Can you work these out from the model? Positions are in its coordinate system, mm. Face numbers are marked on the shaded views. Give positions to 0.01 mm unless a question says otherwise; leave off trailing zeros. Loops run counter-clockwise (first coordinate to the right, second up) from the corner with the lowest first, then second, coordinate; pieces in that order, holes last.
from build123d import *

# Parameters (mm, degrees)
SKETCH_1_W          = 120
SKETCH_1_H          = 135
EXTRUDE_1_DEPTH     = 4
SKETCH_2_W          = 7
SKETCH_2_H          = 95
EXTRUDE_2_DEPTH     = 11
SKETCH_4_R          = 2.35
CUT_EXTRUDE_2_DEPTH = 118.904622471
SKETCH_5_W          = 120
SKETCH_5_H          = 35
CUT_EXTRUDE_3_DEPTH = 10
FILLET_1_R          = 2


with BuildPart() as part:
    # 草图1 → 凸台-拉伸1 (new body)
    with BuildSketch(Plane(origin=(0, 0, 0), x_dir=(1, 0, 0), z_dir=(0, 1, 0))):
        Rectangle(SKETCH_1_W, SKETCH_1_H)
    extrude(amount=EXTRUDE_1_DEPTH)

    # 草图2 → 凸台-拉伸2 (add)
    with BuildSketch(Plane(origin=(0, 4, 0), x_dir=(1, 0, 0), z_dir=(0, 1, 0))):
        with Locations((-32, 20)):
            Rectangle(SKETCH_2_W, SKETCH_2_H)
        with Locations((32, 20)):
            Rectangle(SKETCH_2_W, SKETCH_2_H)
    extrude(amount=EXTRUDE_2_DEPTH)

    # 草图4 → 切除-拉伸2 (cut, through all)
    with BuildSketch(Plane.ZY.offset(35.5)):
        with Locations((20, 9)):
            Circle(SKETCH_4_R)
        with BuildLine():
            Line((-60, 11.35), (-20, 11.35))
            ThreePointArc((-20, 11.35), (-17.65, 9), (-20, 6.65))
            Line((-20, 6.65), (-60, 6.65))
            ThreePointArc((-60, 6.65), (-62.35, 9), (-60, 11.35))
        make_face()
    extrude(amount=-CUT_EXTRUDE_2_DEPTH, mode=Mode.SUBTRACT)

    # 草图5 → 切除-拉伸3 (cut)
    with BuildSketch(Plane(origin=(0, 4, 0), x_dir=(1, 0, 0), z_dir=(0, 1, 0))):
        with Locations((0, -50)):
            Rectangle(SKETCH_5_W, SKETCH_5_H)
    extrude(amount=-CUT_EXTRUDE_3_DEPTH, mode=Mode.SUBTRACT)

    # 圆角1
    fillet_1_edges = [part.edges().sort_by_distance(p)[0] for p in [
        (-35.5, 4, -20),
        (-32, 15, -67.5),
        (-32, 15, 27.5),
        (35.5, 4, -20),
        (32, 15, -67.5),
        (32, 15, 27.5),
        (-60, 2, -67.5),
        (60, 2, -67.5),
        (60, 2, 32.5),
        (-60, 2, 32.5),
    ]]
    fillet(fillet_1_edges, radius=FILLET_1_R)


solid = part.part
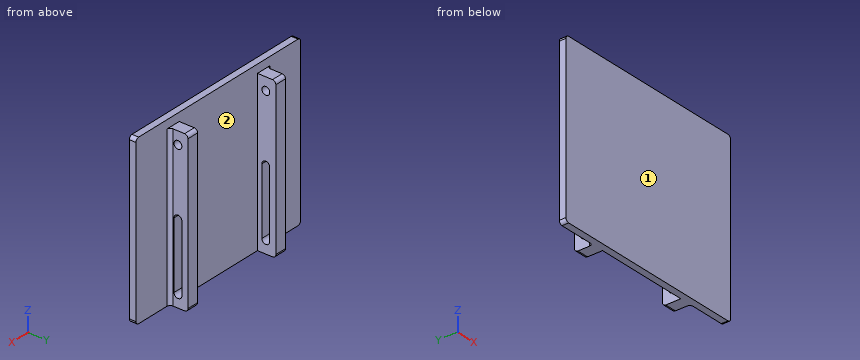
(1) Please list where these lines run through material, in increasing order: probe 1 along Y at (x, z) = (-34, 20); probe 2 along X at (y, z) = (12, -46); probe 3 along Z at (x, y) = (-30, 10).
Returned:
probe 1: y = 0 to 6.65, 11.35 to 15
probe 2: x = -35.5 to -28.5, 28.5 to 35.5
probe 3: z = -67.5 to -62.13, -17.87 to 17.87, 22.13 to 27.5
(2) Suppose I cut it at D-D on x = 27. List the corners of the cut face in (y, z) for me.
Returned:
outline: (0, -67.5) - (4, -67.5) - (4, 32.5) - (0, 32.5) - close
(3) Thinking about a two-plate mould opening in X: for the marked faces 1 and 2, which applies, pulls with the +X half, pulls with the -X half, needs draft (parallel to the pull), parting line crosses it, or undercut?
Returned:
face 1: needs draft
face 2: undercut
(4) Suppose I cut it at C-C on z = 9.5. List the corners of the cut face in (x, y) for me, plus the area to 3 significant figures.
Returned:
outline: (-60, 0) - (60, 0) - (60, 4) - (37.5, 4) arc R2 cw to (35.5, 6) - (35.5, 15) - (28.5, 15) - (28.5, 4) - (-28.5, 4) - (-28.5, 15) - (-35.5, 15) - (-35.5, 6) arc R2 cw to (-37.5, 4) - (-60, 4) - close
area: 636 mm2
(5) Suppose I cut it at B-B on z = 20. List the corners of the cut face in (x, y) for me, plus the area to 3 significant figures.
Returned:
outline: (-60, 0) - (60, 0) - (60, 4) - (37.5, 4) arc R2 cw to (35.5, 6) - (35.5, 6.65) - (28.5, 6.65) - (28.5, 4) - (-28.5, 4) - (-28.5, 6.65) - (-35.5, 6.65) - (-35.5, 6) arc R2 cw to (-37.5, 4) - (-60, 4) - close; (-35.5, 11.35) - (-28.5, 11.35) - (-28.5, 15) - (-35.5, 15) - close; (28.5, 11.35) - (35.5, 11.35) - (35.5, 15) - (28.5, 15) - close
area: 570 mm2
(6) Will these pins go through, and if not, where does the flat tip stop? P1, Ø5.5, axis at y = 9, z = 20, coming from the -X side; P2, Ø7.5, axis at y = 9, z = 20, coming from the -X side; P3, Ø9, axis at y = 10.5, z = -13.5, coming from the +X side.
Returned:
P1: stops at x = -35.5
P2: stops at x = -35.65
P3: stops at x = 35.5
(7) Suppose I cut it at A-A on y = 9. List the corners of the cut face in (x, z) for me.
Returned:
outline: (-35.5, -67.5) - (-28.5, -67.5) - (-28.5, -62.35) - (-35.5, -62.35) - close; (-35.5, -17.65) - (-28.5, -17.65) - (-28.5, 17.65) - (-35.5, 17.65) - close; (-35.5, 22.35) - (-28.5, 22.35) - (-28.5, 27.5) - (-35.5, 27.5) - close; (28.5, -67.5) - (35.5, -67.5) - (35.5, -62.35) - (28.5, -62.35) - close; (28.5, -17.65) - (35.5, -17.65) - (35.5, 17.65) - (28.5, 17.65) - close; (28.5, 22.35) - (35.5, 22.35) - (35.5, 27.5) - (28.5, 27.5) - close
